Verification items for the finished model (mm, model axes). Face numbers are marked on the shaded views. Give positions to 0.01 mm unless a question says otherwise; leave off trailing zeros. Loops run counter-clockwise (first coordinate to the right, second up) from the corner with the lowest first, then second, coordinate; pieces in that order, holes last. Notation, with made-up numbers: (-23.75, 10) - (-2.75, 10) arc R14 cw to (-2.75, 26) - close; hole circle Ø3 at (16, 46). An arc over 180 degrees is marked (long way). Put each result on its own line as item: value. Start each with the question number.
```python
from build123d import *

# Parameters (mm, degrees)
ESBO_O1_W                = 51
ESBO_O1_H                = 51
RESSALTO_EXTRUS_O1_DEPTH = 6
ESBO_O2_W                = 6.5
ESBO_O2_H                = 36.5
CORTE_EXTRUS_O1_DEPTH    = 4.5
ESBO_O3_R                = 2
CORTE_EXTRUS_O2_DEPTH    = 37.558172821
CORTE_EXTRUS_O3_DEPTH    = 4.5
PADR_O_LINEAR1_COUNT     = 3
PADR_O_LINEAR1_PITCH     = 10
FILETE1_R                = 2
CHANFRO1_SIZE            = 1


with BuildPart() as part:
    # Esboço1 → Ressalto-extrusão1 (new body)
    with BuildSketch(Plane.XY):
        Rectangle(ESBO_O1_W, ESBO_O1_H)
    extrude(amount=RESSALTO_EXTRUS_O1_DEPTH)

    # Esboço2 → Corte-extrusão1 (cut)
    with BuildSketch(Plane(origin=(0, 0, 0), x_dir=(-1, 0, 0), z_dir=(0, 0, -1))):
        with Locations((-20.85, -5.85)):
            Rectangle(ESBO_O2_W, ESBO_O2_H)
    extrude(amount=-CORTE_EXTRUS_O1_DEPTH, mode=Mode.SUBTRACT)

    # Esboço3 → Corte-extrusão2 (cut, through all)
    with BuildSketch(Plane.XY.offset(6)):
        with Locations((0, -20.5)):
            Circle(ESBO_O3_R)
        with Locations((0, 20.5)):
            Circle(ESBO_O3_R)
    extrude(amount=-CORTE_EXTRUS_O2_DEPTH, mode=Mode.SUBTRACT)

    # Esboço4 → Corte-extrusão3 (cut)
    with BuildSketch(Plane(origin=(0, 0, 0), x_dir=(-1, 0, 0), z_dir=(0, 0, -1))):
        Polygon((-14.732145215, 17.5), (23.332781841, -0.249966993), (22.064927056, -2.968890354), (-16, 14.781076639), align=None)
    corte_extrus_o3 = extrude(amount=-CORTE_EXTRUS_O3_DEPTH, mode=Mode.SUBTRACT)

    # Padrão linear1: Corte-extrusão3 ×3
    with Locations(*[(0, -i * PADR_O_LINEAR1_PITCH, 0) for i in range(1, PADR_O_LINEAR1_COUNT)]):
        add(corte_extrus_o3, mode=Mode.SUBTRACT)

    # Filete1
    filete1_edges = [part.edges().sort_by_distance(p)[0] for p in [
        (0, 25.5, 6),
    ]]
    fillet(filete1_edges, radius=FILETE1_R)

    # Chanfro1
    chanfro1_edges = [part.edges().sort_by_distance(p)[0] for p in [
        (-2, -20.5, 6),
        (-2, 20.5, 6),
    ]]
    chamfer(chanfro1_edges, length=CHANFRO1_SIZE - 0.0001)  # a hair under: the kernel refuses the full size


solid = part.part
```
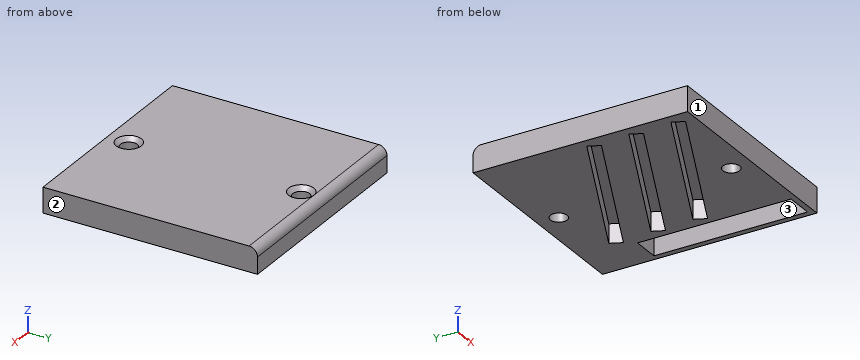
1) Scan lines: line 1 along Y through (x, z) = (0, 2.7); line 2 along Y through (x, z) = (0.5, 4.9); line 3 along Y through (x, z) = (-5.5, 1.75). Record each from-to range of solid material in increasing order. Write a range as from..to.
2) Section check A-A, the plane y = 20.5. Enter the section's corners in (x, z), plus the area to 3 significant figures.
3) Section check B-B, the plane z = 1.75. Enter the section's corners in (x, y).
4) Section check C-C, the plane x = 19. Enter the section's corners in (y, z).
5) Depth check by flat-ended pin: P1, Ø10, axis at x = 6, y = -5.5, coming from the -Z side; P2, Ø2, axis at x = 21, y = 0.5, coming from the -Z side. Enter the tip coordinate at first touch or a pass-through.
6) Section check D-D, the plane x = 0. State how many separate pieces and enclosed holes the cut face has, plus the area to 3 significant figures.
7) Draft check along Y on the marked faces 1, 2 and 3. Enter one of: pulls with the +Y half, pulls with the -Y half, needs draft (parallel to the pull), parting line crosses it, or undercut.
Results are:
1. line 1: y = -25.5..-22.5, -18.5..-12.68, -9.37..-2.68, 0.63..7.32, 10.63..18.5, 22.5..25.5
1. line 2: y = -25.5..-22.44, -18.56..18.56, 22.44..25.29
1. line 3: y = -25.5..-15.24, -11.93..-5.24, -1.93..4.76, 8.07..25.5
2. outline: (-25.5, 0) - (-2, 0) - (-2, 5) - (-3, 6) - (-25.5, 6) - close; (2, 0) - (25.5, 0) - (25.5, 6) - (3, 6) - (2, 5) - close
2. area: 281 mm2
3. outline: (-25.5, -25.5) - (25.5, -25.5) - (25.5, 25.5) - (-25.5, 25.5) - close; hole (-23.33, -20.25) - (-22.06, -22.97) - (16, -5.22) - (14.73, -2.5) - close; hole (-23.33, -10.25) - (-22.06, -12.97) - (16, 4.78) - (14.73, 7.5) - close; hole (-23.33, -0.25) - (-22.06, -2.97) - (16, 14.78) - (14.73, 17.5) - close; hole circle Ø4 at (0, -20.5); hole circle Ø4 at (0, 20.5); hole (17.6, -24.1) - (24.1, -24.1) - (24.1, 12.4) - (17.6, 12.4) - close
4. outline: (-25.5, 0) - (-24.1, 0) - (-24.1, 4.5) - (12.4, 4.5) - (12.4, 0) - (25.5, 0) - (25.5, 4) arc R2 ccw to (23.5, 6) - (-25.5, 6) - close
5. P1: stops at z = 0
5. P2: stops at z = 4.5
6. separate pieces: 3
6. enclosed holes: 0
6. area: 210 mm2
7. face 1: pulls with the -Y half
7. face 2: needs draft
7. face 3: undercut
